Autodesk Inventor part; units mm, degrees
ref_plane "YZ Plane" through (0, 0, 0) normal (1, 0, 0) x (0, 1, 0)
ref_plane "XZ Plane" through (0, 0, 0) normal (0, 1, 0) x (-1, 0, 0)
ref_plane "XY Plane" through (0, 0, 0) normal (0, 0, 1) x (1, 0, 0)
sketch "Sketch1" plane through (0, 0, 0) normal (0, 1, 0) x (-1, 0, 0)
  line L0 (0, 0) -> (40, 0)
  line L1 (40, 0) -> (40, -59)
  line L2 (40, -59) -> (0, -59)
  line L3 (0, -59) -> (0, 0)
  dimension "d0" = 40
  dimension "d1" = 59
extrude "Extrusion1" add sketch "Sketch1" along normal blind 1.57
sketch "Sketch2" plane through (0, 1.57, 0) normal (0, 1, 0) x (1, 0, 0)
  circle A0 centre (-37.5, 1.5) radius 1
  line L0 (-40, 59) -> (-40, 0)
  line L1 (-40, 0) -> (0, 0)
  line L2 (0, 59) -> (-40, 59)
  line L3 (-40, 59) -> (-40, 0)
  line L4 (-40, 0) -> (0, 0)
  line L5 (0, 0) -> (0, 59)
  line L6 (0, 0) -> (0, 59)
  line L7 (0, 59) -> (-40, 59)
  line L8 (0, 29.5) -> (-40, 29.5)
  line L9 (-20, 0) -> (-20, 59)
  circle A1 centre (-37.5, 57.5) radius 1
  circle A2 centre (-2.5, 1.5) radius 1
  circle A3 centre (-2.5, 57.5) radius 1
  dimension "d4" = 2
  dimension "d5" = 2.5
  dimension "d6" = 1.5
extrude "Extrusion2" cut sketch "Sketch2" against normal blind 2 contours A0 | A1 | A2 | A3
equation "\"d7\" = d4"
properties part number "pcb sola" material "Steel, Mild, Welded"
For this review, take the finished solid that the model builds, in its own axes (mm). Round coordinates to 2 decimals unless told otherwise and drop trailing zeros. Loops run counter-clockwise (first coordinate to the right, second up) from the corner with the lowest first, then second, coordinate; pieces in that order, holes last. Notation, with made-up numbers: (55.25, 51.25) - (69.25, 51.25) arc R9 cw to (69.25, 64.25) - close; hole circle Ø10 at (51.5, 25.25). An arc over 180 degrees is marked (long way). One line per question, with ' | ' between items.
Q1. For line 1 along X through (y, z) = (1.2, -1.5); line 2 along Z through (x, y) = (-37.5, 0.95), list the stretches that pass through material, from the lowest coordinate up. Write a range as [from, to].
Taken from the geometry:
line 1: x = [-40, -38.5], [-36.5, -3.5], [-1.5, 0] | line 2: z = [-59, -58.5], [-56.5, -2.5], [-0.5, 0]
Q2. Take a section at A-A (x = -2.5). Give the boundary of the cut face in (y, z).
Taken from the geometry:
outline: (0, -59) - (1.57, -59) - (1.57, -58.5) - (0, -58.5) - close; (0, -56.5) - (1.57, -56.5) - (1.57, -2.5) - (0, -2.5) - close; (0, -0.5) - (1.57, -0.5) - (1.57, 0) - (0, 0) - close
Q3. The part is to be moulded in two halves that separate along Z. For faces 1 (the cylindrical face through (-3.3, 0.8, -0.9)), 2 (the cylindrical face through (-1.96, 0.8, -58.34)), 3 (the flat face through (-20, 1.57, -29)), 4 (the flat face through (-20, 1, -59)), say which applies: released by +Z, released by -Z, zero draft, split by the parting line, or undercut.
Taken from the geometry:
face 1: undercut | face 2: undercut | face 3: zero draft | face 4: released by -Z
Q4. For pin 1 (1.2 mm diameter, centred on x = -37.5, z = -57.5, fed in from +Y), flat-tipped, find the tip position at first contact; note if it passes through.
Taken from the geometry:
pin 1: passes through
Q5. Take a section at B-B (z = -57.5). Give the boundary of the cut face in (x, y).
Taken from the geometry:
outline: (-40, 0) - (-38.5, 0) - (-38.5, 1.57) - (-40, 1.57) - close; (-36.5, 0) - (-3.5, 0) - (-3.5, 1.57) - (-36.5, 1.57) - close; (-1.5, 0) - (0, 0) - (0, 1.57) - (-1.5, 1.57) - close
